The model under review builds one solid part; all positions refer to its coordinate system, in mm. Face numbers are marked on the shaded views. A direction names the side the tool comes from. Round coordinates to 2 decimals unless told otherwise and drop trailing zeros. Order: outer loops, then holes, each group sorted by start corner. A loop starts at its lowest first (then second) coordinate and runs counter-clockwise, first axis right, second up. Notation, with made-up numbers: M 73.25,40 L 85.25,40 A17 ccw 85.25,55 Z; hole C 37.25,19.5 d10. An arc over 180 degrees is marked long. Use a Markdown table: item, result. Add a question column.
1. Consider section D-D on y = 35.5. State the section outline as (x, z) points, then the cut area to 3 significant figures.
2. For the marked faces 1, 2 and 3, list the 3-axis set-ups (+Z, -Z, +X, -X, +Y, -Y) from which the entire face can be reached by the end or side of a thin tool; tool diameter is ignored.
3. To check wall thickness, follow probe 1 along Y at (x, z) = (5, 11); probe 2 along Y at (x, z) = (22, 17); probe 3 along X at (y, z) = (-1.5, 8). State the ranges of each line that lie inside material, in increasing order.
4. Consider section B-B on z = 24. State the section outline as (x, y) points.
5. Consider section A-A on y = -1. State the section outline as (x, z) points.
6. The part is to be moulded in two halves that separate along X. For the marked faces 4, 5 and 6, say which applies: +X half, -X half, draft (parallel to the pull), parting line (faces both ways), or undercut.
7. Insertion check: P1, Ø5, axis at x = 21, y = 34, coming from the +Z side; P2, Ø4, axis at y = 11.5, z = 26.5, coming from the -X side; P3, Ø10, axis at x = 2.5, y = 4.5, coming from the -Z side; P4, Ø2.5, axis at x = -5, z = 14.5, coming from the +Y side. Each pin has a flat end and moves straight along its axis. Give the tip position at first contact, or say it passes through.
8. Consider section C-C on x = 12. State the section outline as (y, z) points.
from build123d import *

# Parameters (mm, degrees)
BOX010_W                = 22
BOX010_H                = 10
BOX010_DEPTH            = 10
BOX010_ROLL_ANGLE       = 45
BOX009_W                = 22
BOX009_H                = 10
BOX009_DEPTH            = 10
BOX009_ROLL_ANGLE       = 45
CYLINDER010_R           = 1.5
CYLINDER010_DEPTH       = 40
CYLINDER010_PITCH_ANGLE = 90
CYLINDER011_R           = 1.5
CYLINDER011_DEPTH       = 40
CYLINDER011_PITCH_ANGLE = 90
CYLINDER012_R           = 1.5
CYLINDER012_DEPTH       = 40
CYLINDER012_PITCH_ANGLE = 90
CYLINDER009_R           = 1.5
CYLINDER009_DEPTH       = 40
CYLINDER009_PITCH_ANGLE = 90
BOX004_W                = 2
BOX004_H                = 32
BOX004_DEPTH            = 6
CYLINDER_R              = 13
CYLINDER_DEPTH          = 25
CYLINDER001_R           = 13.5
CYLINDER001_DEPTH       = 18
CYLINDER001_PITCH_ANGLE = 90
CYLINDER003_R           = 1.4
CYLINDER003_DEPTH       = 20
CYLINDER003_PITCH_ANGLE = 90
CYLINDER005_R           = 1.4
CYLINDER005_DEPTH       = 20
CYLINDER005_PITCH_ANGLE = 90
CYLINDER004_R           = 1.4
CYLINDER004_DEPTH       = 20
CYLINDER004_PITCH_ANGLE = 90
CYLINDER002_R           = 1.4
CYLINDER002_DEPTH       = 20
CYLINDER002_PITCH_ANGLE = 90
BOX002_W                = 6
BOX002_H                = 7
BOX002_DEPTH            = 20
BOX006_W                = 4.5
BOX006_H                = 7
BOX006_DEPTH            = 16
BOX007_W                = 4.5
BOX007_H                = 7
BOX007_DEPTH            = 16
BOX008_W                = 4.5
BOX008_H                = 7
BOX008_DEPTH            = 16
BOX005_W                = 4.5
BOX005_H                = 7
BOX005_DEPTH            = 16
BOX003_W                = 6
BOX003_H                = 7
BOX003_DEPTH            = 20
BOX001_W                = 6
BOX001_H                = 32
BOX001_DEPTH            = 30
BOX_W                   = 24
BOX_H                   = 32
BOX_DEPTH               = 25
FILLET_R                = 4
FILLET001_R             = 4
FILLET002_R             = 4
FILLET003_R             = 4


with BuildPart() as cube010:
    # Box010 → Box010 (new body)
    with BuildSketch(Plane.XY):
        with Locations((11, 5)):
            Rectangle(BOX010_W, BOX010_H)
    extrude(amount=BOX010_DEPTH)


with BuildPart() as cube010_1:
    # Box010 roll: moved
    add(cube010.part.rotate(Axis((0, 0, 0), (1, 0, 0)), BOX010_ROLL_ANGLE))


with BuildPart() as cube010_2:
    # Box010 placement: moved
    add(cube010_1.part.moved(Location((2, 41, -7))))


with BuildPart() as fusionwingcuts:
    # Box009 → Box009 (new body)
    with BuildSketch(Plane.XY):
        with Locations((11, 5)):
            Rectangle(BOX009_W, BOX009_H)
    extrude(amount=BOX009_DEPTH)


with BuildPart() as fusionwingcuts_1:
    # Box009 roll: moved
    add(fusionwingcuts.part.rotate(Axis((0, 0, 0), (1, 0, 0)), BOX009_ROLL_ANGLE))


with BuildPart() as fusionwingcuts_2:
    # Box009 placement: moved
    add(fusionwingcuts_1.part.moved(Location((2, -9, -7))))

    # Fusion005: union Cube010
    add(cube010_2.part)


with BuildPart() as fusionwingcuts_3:
    # Fusion005 placement: moved
    add(fusionwingcuts_2.part.moved(Location((0, 0, 5.5))))


with BuildPart() as cylinder010:
    # Cylinder010 → Cylinder010 (new body)
    with BuildSketch(Plane.XY):
        Circle(CYLINDER010_R)
    extrude(amount=CYLINDER010_DEPTH)


with BuildPart() as cylinder010_1:
    # Cylinder010 pitch: moved
    add(cylinder010.part.rotate(Axis((0, 0, 0), (0, 1, 0)), CYLINDER010_PITCH_ANGLE))


with BuildPart() as cylinder010_2:
    # Cylinder010 placement: moved
    add(cylinder010_1.part.moved(Location((0, -3.5, 6))))


with BuildPart() as cylinder011:
    # Cylinder011 → Cylinder011 (new body)
    with BuildSketch(Plane.XY):
        Circle(CYLINDER011_R)
    extrude(amount=CYLINDER011_DEPTH)


with BuildPart() as cylinder011_1:
    # Cylinder011 pitch: moved
    add(cylinder011.part.rotate(Axis((0, 0, 0), (0, 1, 0)), CYLINDER011_PITCH_ANGLE))


with BuildPart() as cylinder011_2:
    # Cylinder011 placement: moved
    add(cylinder011_1.part.moved(Location((0, 35.5, 12))))


with BuildPart() as cylinder012:
    # Cylinder012 → Cylinder012 (new body)
    with BuildSketch(Plane.XY):
        Circle(CYLINDER012_R)
    extrude(amount=CYLINDER012_DEPTH)


with BuildPart() as cylinder012_1:
    # Cylinder012 pitch: moved
    add(cylinder012.part.rotate(Axis((0, 0, 0), (0, 1, 0)), CYLINDER012_PITCH_ANGLE))


with BuildPart() as cylinder012_2:
    # Cylinder012 placement: moved
    add(cylinder012_1.part.moved(Location((0, 35.5, 6))))


with BuildPart() as fusionwingscrews:
    # Cylinder009 → Cylinder009 (new body)
    with BuildSketch(Plane.XY):
        Circle(CYLINDER009_R)
    extrude(amount=CYLINDER009_DEPTH)


with BuildPart() as fusionwingscrews_1:
    # Cylinder009 pitch: moved
    add(fusionwingscrews.part.rotate(Axis((0, 0, 0), (0, 1, 0)), CYLINDER009_PITCH_ANGLE))


with BuildPart() as fusionwingscrews_2:
    # Cylinder009 placement: moved
    add(fusionwingscrews_1.part.moved(Location((0, -3.5, 12))))

    # Fusion004: union Cylinder010, Cylinder011, Cylinder012
    add(cylinder010_2.part)
    add(cylinder011_2.part)
    add(cylinder012_2.part)


with BuildPart() as fusionwingscrews_3:
    # Fusion004 placement: moved
    add(fusionwingscrews_2.part.moved(Location((0, 0, 5.5))))


with BuildPart() as obj1:
    # Box004 → Box004 (new body)
    with BuildSketch(Plane(origin=(-4, 0, 10), x_dir=(1, 0, 0), z_dir=(0, 0, 1))):
        with Locations((1, 16)):
            Rectangle(BOX004_W, BOX004_H)
    extrude(amount=BOX004_DEPTH)


with BuildPart() as cylinderheatsink:
    # Cylinder → Cylinder (new body)
    with BuildSketch(Plane(origin=(6.4, 16, 0), x_dir=(1, 0, 0), z_dir=(0, 0, 1))):
        Circle(CYLINDER_R)
    extrude(amount=CYLINDER_DEPTH)


with BuildPart() as cylinderfan:
    # Cylinder001 → Cylinder001 (new body)
    with BuildSketch(Plane.XY):
        Circle(CYLINDER001_R)
    extrude(amount=CYLINDER001_DEPTH)


with BuildPart() as cylinderfan_1:
    # Cylinder001 pitch: moved
    add(cylinderfan.part.rotate(Axis((0, 0, 0), (0, 1, 0)), CYLINDER001_PITCH_ANGLE))


with BuildPart() as cylinderfan_2:
    # Cylinder001 placement: moved
    add(cylinderfan_1.part.moved(Location((13, 16, 15))))


with BuildPart() as obj2:
    # Cylinder003 → Cylinder003 (new body)
    with BuildSketch(Plane.XY):
        Circle(CYLINDER003_R)
    extrude(amount=CYLINDER003_DEPTH)


with BuildPart() as obj2_1:
    # Cylinder003 pitch: moved
    add(obj2.part.rotate(Axis((0, 0, 0), (0, 1, 0)), CYLINDER003_PITCH_ANGLE))


with BuildPart() as obj2_2:
    # Cylinder003 placement: moved
    add(obj2_1.part.moved(Location((20, 4, 27))))


with BuildPart() as obj3:
    # Cylinder005 → Cylinder005 (new body)
    with BuildSketch(Plane.XY):
        Circle(CYLINDER005_R)
    extrude(amount=CYLINDER005_DEPTH)


with BuildPart() as obj3_1:
    # Cylinder005 pitch: moved
    add(obj3.part.rotate(Axis((0, 0, 0), (0, 1, 0)), CYLINDER005_PITCH_ANGLE))


with BuildPart() as obj3_2:
    # Cylinder005 placement: moved
    add(obj3_1.part.moved(Location((20, 28, 3))))


with BuildPart() as obj4:
    # Cylinder004 → Cylinder004 (new body)
    with BuildSketch(Plane.XY):
        Circle(CYLINDER004_R)
    extrude(amount=CYLINDER004_DEPTH)


with BuildPart() as obj4_1:
    # Cylinder004 pitch: moved
    add(obj4.part.rotate(Axis((0, 0, 0), (0, 1, 0)), CYLINDER004_PITCH_ANGLE))


with BuildPart() as obj4_2:
    # Cylinder004 placement: moved
    add(obj4_1.part.moved(Location((20, 28, 27))))


with BuildPart() as fusioncuts:
    # Cylinder002 → Cylinder002 (new body)
    with BuildSketch(Plane.XY):
        Circle(CYLINDER002_R)
    extrude(amount=CYLINDER002_DEPTH)


with BuildPart() as fusioncuts_1:
    # Cylinder002 pitch: moved
    add(fusioncuts.part.rotate(Axis((0, 0, 0), (0, 1, 0)), CYLINDER002_PITCH_ANGLE))


with BuildPart() as fusioncuts_2:
    # Cylinder002 placement: moved
    add(fusioncuts_1.part.moved(Location((20, 4, 3))))

    # Fusion001: union obj2, obj3, obj4
    add(obj2_2.part)
    add(obj3_2.part)
    add(obj4_2.part)

    # Fusion: union FusionWingCuts, FusionWingScrews, obj1, CylinderHeatSink, CylinderFan
    add(fusionwingcuts_3.part)
    add(fusionwingscrews_3.part)
    add(obj1.part)
    add(cylinderheatsink.part)
    add(cylinderfan_2.part)


with BuildPart() as obj5:
    # Box002 → Box002 (new body)
    with BuildSketch(Plane(origin=(-6, 0, 0), x_dir=(1, 0, 0), z_dir=(0, 0, 1))):
        with Locations((3, 3.5)):
            Rectangle(BOX002_W, BOX002_H)
    extrude(amount=BOX002_DEPTH)


with BuildPart() as cube006:
    # Box006 → Box006 (new body)
    with BuildSketch(Plane(origin=(19, -7, 0), x_dir=(1, 0, 0), z_dir=(0, 0, 1))):
        with Locations((2.25, 3.5)):
            Rectangle(BOX006_W, BOX006_H)
    extrude(amount=BOX006_DEPTH)


with BuildPart() as cube007:
    # Box007 → Box007 (new body)
    with BuildSketch(Plane(origin=(2, 32, 0), x_dir=(1, 0, 0), z_dir=(0, 0, 1))):
        with Locations((2.25, 3.5)):
            Rectangle(BOX007_W, BOX007_H)
    extrude(amount=BOX007_DEPTH)


with BuildPart() as cube008:
    # Box008 → Box008 (new body)
    with BuildSketch(Plane(origin=(19, 32, 0), x_dir=(1, 0, 0), z_dir=(0, 0, 1))):
        with Locations((2.25, 3.5)):
            Rectangle(BOX008_W, BOX008_H)
    extrude(amount=BOX008_DEPTH)


with BuildPart() as fusionwings:
    # Box005 → Box005 (new body)
    with BuildSketch(Plane(origin=(2, -7, 0), x_dir=(1, 0, 0), z_dir=(0, 0, 1))):
        with Locations((2.25, 3.5)):
            Rectangle(BOX005_W, BOX005_H)
    extrude(amount=BOX005_DEPTH)

    # Fusion006: union Cube006, Cube007, Cube008
    add(cube006.part)
    add(cube007.part)
    add(cube008.part)


with BuildPart() as fusionwings_1:
    # Fusion006 placement: moved
    add(fusionwings.part.moved(Location((0, 0, 5.5))))


with BuildPart() as obj6:
    # Box003 → Box003 (new body)
    with BuildSketch(Plane(origin=(-6, 25, 0), x_dir=(1, 0, 0), z_dir=(0, 0, 1))):
        with Locations((3, 3.5)):
            Rectangle(BOX003_W, BOX003_H)
    extrude(amount=BOX003_DEPTH)


with BuildPart() as obj7:
    # Box001 → Box001 (new body)
    with BuildSketch(Plane(origin=(24, 0, 0), x_dir=(1, 0, 0), z_dir=(0, 0, 1))):
        with Locations((3, 16)):
            Rectangle(BOX001_W, BOX001_H)
    extrude(amount=BOX001_DEPTH)


with BuildPart() as obj8:
    # Box → Box (new body)
    with BuildSketch(Plane.XY):
        with Locations((12, 16)):
            Rectangle(BOX_W, BOX_H)
    extrude(amount=BOX_DEPTH)

    # Fusion007: union obj5, FusionWings, obj6, obj7
    add(obj5.part)
    add(fusionwings_1.part)
    add(obj6.part)
    add(obj7.part)

    # Fillet
    fillet_edges = [obj8.edges().sort_by_distance(p)[0] for p in [
        (-6, 3.5, 0),
    ]]
    fillet(fillet_edges, radius=FILLET_R)

    # Fillet001
    fillet001_edges = [obj8.edges().sort_by_distance(p)[0] for p in [
        (12, 0, 0),
    ]]
    fillet(fillet001_edges, radius=FILLET001_R)

    # Fillet002
    fillet002_edges = [obj8.edges().sort_by_distance(p)[0] for p in [
        (12, 32, 0),
    ]]
    fillet(fillet002_edges, radius=FILLET002_R)

    # Fillet003
    fillet003_edges = [obj8.edges().sort_by_distance(p)[0] for p in [
        (-6, 26.5, 0),
    ]]
    fillet(fillet003_edges, radius=FILLET003_R)

    # Cut: cut FusionCUTS
    add(fusioncuts_2.part, mode=Mode.SUBTRACT)


solid = obj8.part
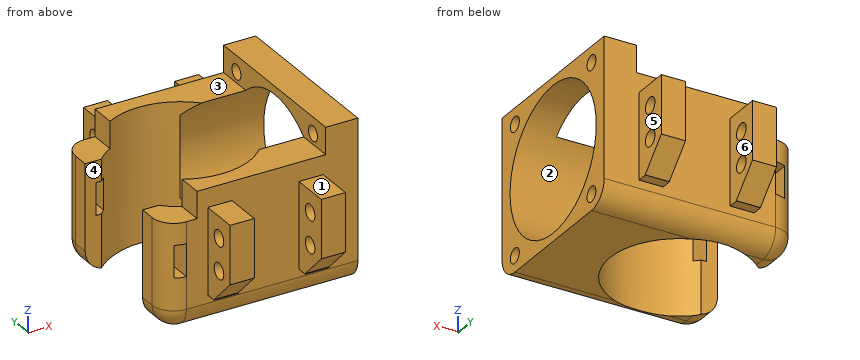
Answer block:
| question | item | result |
|---|---|---|
| 1 | outline | M 2,7.14 L 6.5,7.14 L 6.5,10 L 2,10 Z; M 2,13 L 6.5,13 L 6.5,16 L 2,16 Z; M 2,19 L 6.5,19 L 6.5,21.5 L 2,21.5 Z; M 19,7.14 L 23.5,7.14 L 23.5,10 L 19,10 Z; M 19,13 L 23.5,13 L 23.5,16 L 19,16 Z; M 19,19 L 23.5,19 L 23.5,21.5 L 19,21.5 Z |
| 1 | area | 75.2 mm^2 |
| 2 | face 1 | +Z, +X, -X, -Y |
| 2 | face 2 | +X |
| 2 | face 3 | +Z, -X, +Y, -Y |
| 3 | probe 1 | -7 to -4.91, -2.09 to 3.08, 28.92 to 34.09, 36.91 to 39 |
| 3 | probe 2 | -7 to -4.91, -2.09 to 2.65, 29.35 to 34.09, 36.91 to 39 |
| 3 | probe 3 | 2 to 6.5, 19 to 23.5 |
| 4 | outline | M 0,0 L 30,0 L 30,5.94 L 14.63,5.94 A13 cw 0,4.68 Z; M 0,27.32 A13 cw 14.63,26.06 L 30,26.06 L 30,32 L 0,32 Z |
| 5 | outline | M 2,5.5 L 6.5,5.5 L 6.5,21.5 L 2,21.5 Z; M 19,5.5 L 23.5,5.5 L 23.5,21.5 L 19,21.5 Z |
| 6 | face 4 | draft |
| 6 | face 5 | +X half |
| 6 | face 6 | undercut |
| 7 | P1 | z = 25 |
| 7 | P2 | x = 24 |
| 7 | P3 | z = 0 |
| 7 | P4 | y = 31.46 |
| 8 | outline | M 0,4 A4 ccw 4,0 L 4.27,0 L 4.27,25 L 0,25 Z; M 27.73,0 L 28,0 A4 ccw 32,4 L 32,25 L 27.73,25 Z |
